Here's how the part is built. I have some questions about the finished solid (model axes, mm). Face numbers are marked on the shaded views. A direction names the side the tool comes from. Coordinates: 2 decimals unless noted, no trailing zeros. Write each loop counter-clockwise with the first axis right and the second up, starting at its lowest first coordinate (ties: lowest second). Pieces come first, ordered by that corner, then holes.
from build123d import *

# Parameters (mm, degrees)
ESBO_O1_R                = 1.5
RESSALTO_EXTRUS_O1_DEPTH = 4
ESBO_O2_W                = 23
ESBO_O2_H                = 12
ESBO_O2_R                = 2.5
RESSALTO_EXTRUS_O2_DEPTH = 4
FILETE1_R                = 3


with BuildPart() as part:
    # Esboço1 → Ressalto-extrusão1 (new body)
    with BuildSketch(Plane(origin=(0, 0, 0), x_dir=(1, 0, 0), z_dir=(0, 1, 0))):
        Polygon((-3.5, 0), (3.5, 0), (3.5, 10), (11.5, 10), (11.5, -4), (-11.5, -4), (-11.5, 10), (-3.5, 10), align=None)
        with Locations((-7.5, 6)):
            Circle(ESBO_O1_R, mode=Mode.SUBTRACT)
        with Locations((7.5, 6)):
            Circle(ESBO_O1_R, mode=Mode.SUBTRACT)
    extrude(amount=RESSALTO_EXTRUS_O1_DEPTH)

    # Esboço2 → Ressalto-extrusão2 (add)
    with BuildSketch(Plane.XY.offset(4)):
        with Locations((0, -6)):
            Rectangle(ESBO_O2_W, ESBO_O2_H)
        with Locations((0, -6)):
            Circle(ESBO_O2_R, mode=Mode.SUBTRACT)
    extrude(amount=-RESSALTO_EXTRUS_O2_DEPTH)

    # Filete1
    filete1_edges = [part.edges().sort_by_distance(p)[0] for p in [
        (-3.5, 2, 0),
        (3.5, 2, 0),
        (3.5, 2, -10),
        (11.5, 2, -10),
        (-11.5, 2, -10),
        (-3.5, 2, -10),
        (-7.5, 0, 0),
        (11.5, -12, 2),
        (-11.5, -12, 2),
        (7.5, 0, 0),
    ]]
    fillet(filete1_edges, radius=FILETE1_R)


solid = part.part
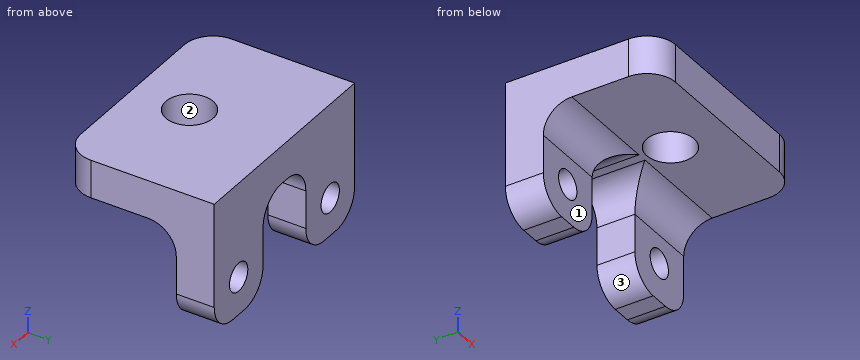
1. On a 3-axis mill with a long thin cutter (end or side, diameter ignored), from which of +Z, -Z, +X, -X, +Y, -Y can I reach the whole of each face in a straight line? I mean the marked faces 1, 2 and 3. Say none if no direction works.
2. I want a section at A-A (y = -8). List the corners of the cut face in (x, z) for me, then the cut area to 3 significant figures.
3. I want a section at D-D (x = 7.5). List the corners of the cut face in (y, z) for me, then the cut area to 3 significant figures.
4. For pin 1 Ø3.5 at (x, z) = (-7, -7.5) entering from -Y; pin 2 Ø4 at (x, y) = (0, -6) entering from +Z; pin 3 Ø1.5 at (y, z) = (-0.5, -5) entering from +X; pin 4 Ø1 at (x, z) = (7, -2) entering from -Y, each with a flat end and sliding along its axis, tell me the tip position at first contact or that it passes through.
5. I want a section at B-B (z = -3.75). List the corners of the cut face in (x, y) for me, then the cut area to 3 significant figures.
6. I want a section at C-C (z = -6). List the corners of the cut face in (x, y) for me.
7. If I drill on line 1 (X direction, y = 1.4, z = -6); line 2 (Y direction, x = 0, z = 1); line 3 (Y direction, x = 7.5, z = -4.25), over which ranges is the centre line in solid material (lowest first)?
Response values:
1. face 1: -Z, +X, -X, -Y
1. face 2: +Z, -Z
1. face 3: -Z, +Y, -Y
2. outline: (-11.5, 0) - (-1.5, 0) - (-1.5, 4) - (-11.5, 4) - close; (1.5, 0) - (11.5, 0) - (11.5, 4) - (1.5, 4) - close
2. area: 80.0 mm2
3. outline: (-12, 0) - (-3, 0) arc R3 cw to (0, -3) - (0, -4.5) - (4, -4.5) - (4, 4) - (-12, 4) - close; (0, -10) - (4, -10) - (4, -7.5) - (0, -7.5) - close
3. area: 93.9 mm2
4. pin 1: stops at y = 0
4. pin 2: passes through
4. pin 3: stops at x = 11.5
4. pin 4: stops at y = -0.4
5. outline: (-11.5, 0) - (-3.5, 0) - (-3.5, 4) - (-11.5, 4) - close; (3.5, 0) - (11.5, 0) - (11.5, 4) - (3.5, 4) - close
5. area: 64.0 mm2
6. outline: (-11.5, 0) - (-9, 0) - (-9, 4) - (-11.5, 4) - close; (-6, 0) - (-3.5, 0) - (-3.5, 4) - (-6, 4) - close; (3.5, 0) - (6, 0) - (6, 4) - (3.5, 4) - close; (9, 0) - (11.5, 0) - (11.5, 4) - (9, 4) - close
7. line 1: x = -11.5 to -9, -6 to -3.5, 3.5 to 6, 9 to 11.5
7. line 2: y = -12 to -8.5, -3.5 to 4
7. line 3: y = 0 to 4
